Here's the drawing with two shaded views (mm, measured from the low corner). I have some questions. A direction names the side the tool comes from. Coordinates: 2 decimals unless noted, no trailing zeros. Order: outer loops, then holes, each group sorted by start corner. A loop starts at its lowest first (then second) coordinate and runs counter-clockwise, first axis right, second up. Notation, with made-up numbers: (72.5, 14.5) -> (111.5, 14.5) arc R30 cw to (111.5, 44.5) -> close; hole circle Ø9 at (-11, 19). An arc over 180 degrees is marked (long way). Return JSON: item names as keys, results as strings. Group by question number.
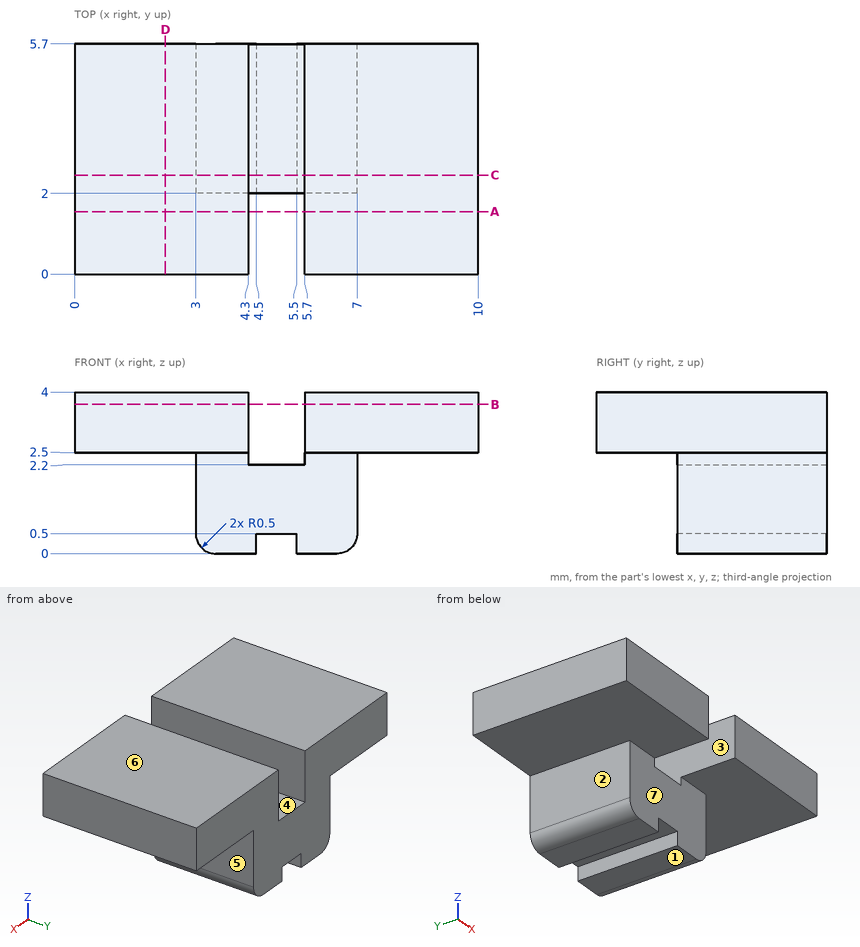
Q1. I'm going to push flat-ended pins straight in: pin 1 Ø1 at (x, y) = (4, 3) entering from -Z; pin 2 Ø0.6 at (y, z) = (3.5, 1) entering from +X; pin 3 Ø0.7 at (x, y) = (5, 4) entering from +Z; pin 4 Ø2 at (x, z) = (5, 1.5) entering from -Y. Where does each tip first touch, or does it pass through?
Q2. We'd pull the mould along X, two halves only. Please class the marked faces 1, 2 and 3: pulls with the +X half, pulls with the -X half, needs draft (parallel to the pull), parting line crosses it, or undercut.
Q3. I want a section at D-D on x = 2.25. Please give me the cut outline in (y, z).
Q4. On a 3-axis mill with a long thin cutter (end or side, diameter ignored), from which of +Z, -Z, +X, -X, +Y, -Y can I reach the whole of each face in a straight line? I mean the marked faces 4, 5, 6 and 7. Say none if no direction works.
Q5. I need wall thicknesses on line 1 along X through (y, z) = (3.4, 3.35); line 2 along Z through (x, y) = (0.5, 1); line 3 along Y through (x, z) = (4, 0.7). Which ranges of each line are inside material? Lowest first, please. Write a range as from..to.
Q6. I want a section at A-A on y = 1.55. Please give me the cut outline in (x, z).
Q7. I want a section at C-C on y = 2.45. Please give me the cut outline in (x, z).
Q8. I want a section at B-B on z = 3.7. Please give me the cut outline in (x, y), and give its area (3 significant figures).
Response values:
{
 "1": {"pin 1": "stops at z = 0", "pin 2": "stops at x = 7", "pin 3": "stops at z = 2.2", "pin 4": "stops at y = 2"},
 "2": {"face 1": "needs draft", "face 2": "pulls with the -X half", "face 3": "undercut"},
 "3": {"outline": "(0, 2.5) -> (5.7, 2.5) -> (5.7, 4) -> (0, 4) -> close"},
 "4": {"face 4": "+Z, +Y, -Y", "face 5": "-Z, +X, +Y, -Y", "face 6": "+Z, +X, -X, +Y, -Y", "face 7": "-Z, +X, -X, -Y"},
 "5": {"line 1": "x = 0..4.3, 5.7..10", "line 2": "z = 2.5..4", "line 3": "y = 2..5.7"},
 "6": {"outline": "(0, 2.5) -> (4.3, 2.5) -> (4.3, 4) -> (0, 4) -> close; (5.7, 2.5) -> (10, 2.5) -> (10, 4) -> (5.7, 4) -> close"},
 "7": {"outline": "(0, 2.5) -> (3, 2.5) -> (3, 0.5) arc R0.5 ccw to (3.5, 0) -> (4.5, 0) -> (4.5, 0.5) -> (5.5, 0.5) -> (5.5, 0) -> (6.5, 0) arc R0.5 ccw to (7, 0.5) -> (7, 2.5) -> (10, 2.5) -> (10, 4) -> (5.7, 4) -> (5.7, 2.2) -> (4.3, 2.2) -> (4.3, 4) -> (0, 4) -> close"},
 "8": {"outline": "(0, 0) -> (4.3, 0) -> (4.3, 5.7) -> (0, 5.7) -> close; (5.7, 0) -> (10, 0) -> (10, 5.7) -> (5.7, 5.7) -> close", "area": "49.0 mm²"}
}
